Answer from the drawing. Dimensions are ordinates in mm from the lowest x, y and z of the part. A direction names the side the tool comes from. Give positions to 0.01 mm unless a question says otherwise; leave off trailing zeros. Loops run counter-clockwise (first coordinate to the right, second up) from the corner with the lowest first, then second, coordinate; pieces in that order, holes last. Notation, with made-up numbers: M 15.25,17.5 L 27.25,17.5 A22 ccw 27.25,53.5 Z; hole C 41.25,57 d1. An arc over 180 degrees is marked long. Use a Markdown table: item, result.
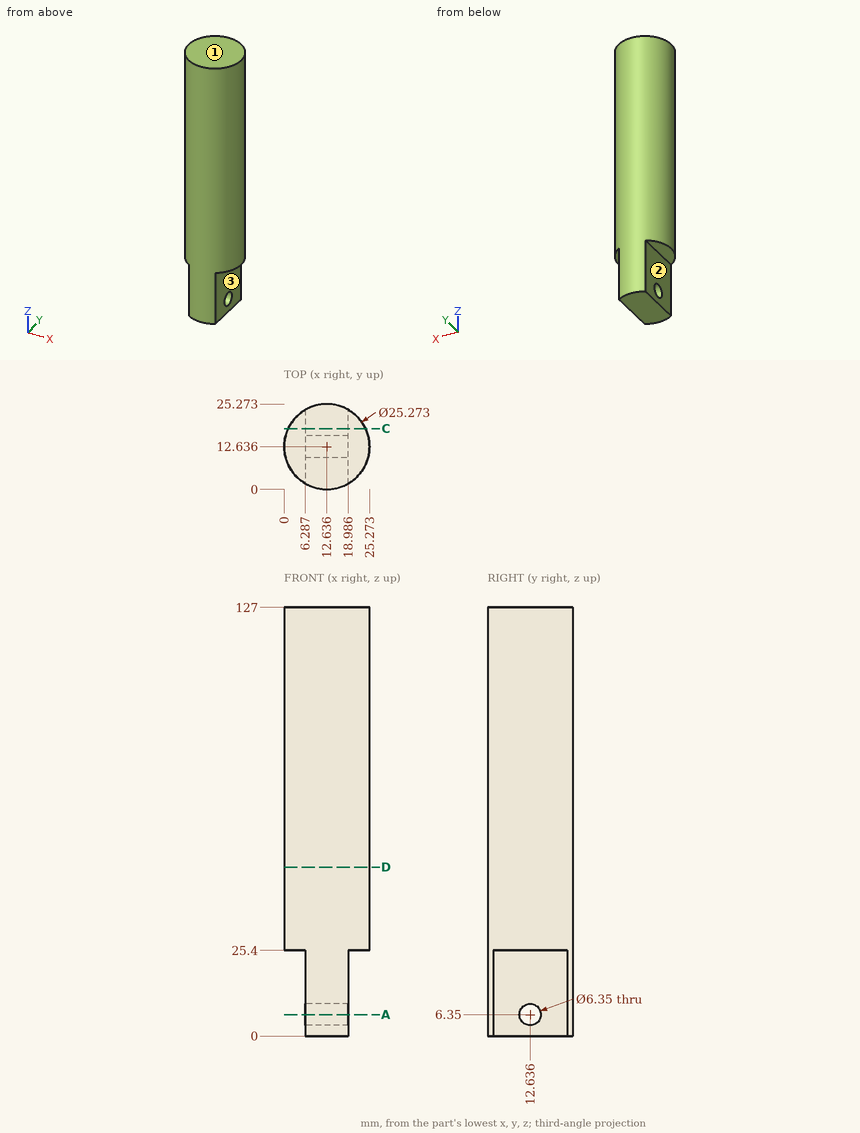
(1) Given P1, Ø1.9, axis at x = 4, y = 14.5, coming from the -Z side; P2, Ø11, axis at y = 11, z = 16.5, coming from the +X side; P3, Ø10, axis at y = 2.5, z = 28.5, coming from the +X side; P4, Ø5.5, axis at y = 12.64, z = 6.35, coming from the -X side, each flat-ended and moving along its own axis, determine where each tip first touches the part or whether it passes through.
Entries:
| item | result |
|---|---|
| P1 | stops at z = 25.4 |
| P2 | stops at x = 18.99 |
| P3 | stops at x = 24.18 |
| P4 | passes through |
(2) A cutting plane is placed at A-A (z = 6.35). Write down the section's boundary in (x, y), and give its area (3 significant figures).
Entries:
| item | result |
|---|---|
| outline | M 6.29,1.71 A12.64 ccw 18.99,1.71 L 18.99,9.46 L 6.29,9.46 Z; M 6.29,15.81 L 18.99,15.81 L 18.99,23.56 A12.64 ccw 6.29,23.56 Z |
| area | 226 mm² |
(3) Consider probe 1 along X at (y, z) = (18, 18); probe 2 along Z at (x, y) = (3.5, 9.75); probe 3 along X at (y, z) = (12.25, 34.5) (1 decimal). Determine where each line is inside the solid, lowest interval first. Write a range as [from, to].
Entries:
| item | result |
|---|---|
| probe 1 | x = [6.29, 18.99] |
| probe 2 | z = [25.4, 127] |
| probe 3 | x = [0, 25.3] |
(4) Which of the six approach directions +Z, -Z, +X, -X, +Y, -Y give full straight-line access (tool end or side, diameter ignored) to the marked faces 1, 2 and 3?
Entries:
| item | result |
|---|---|
| face 1 | +Z, +X, -X, +Y, -Y |
| face 2 | -Z, -X, +Y, -Y |
| face 3 | -Z, +X, +Y, -Y |
(5) A cutting plane is placed at C-C (y = 18). Write down the section's boundary in (x, z) (1 decimal).
Entries:
| item | result |
|---|---|
| outline | M 1.2,25.4 L 6.3,25.4 L 6.3,0 L 19,0 L 19,25.4 L 24.1,25.4 L 24.1,127 L 1.2,127 Z |
(6) A cutting plane is placed at D-D (z = 50). Write down the section's boundary in (x, y).
Entries:
| item | result |
|---|---|
| outline | C 12.64,12.64 d25.27 |
